Part model, mm, in its own coordinate system. Face numbers are marked on the shaded views. A direction names the side the tool comes from. Round coordinates to 2 decimals unless told otherwise and drop trailing zeros. Order: outer loops, then holes, each group sorted by start corner. A loop starts at its lowest first (then second) coordinate and runs counter-clockwise, first axis right, second up. Notation, with made-up numbers: (53, 73) - (61, 73) arc R28 ccw to (61, 112) - close; hole circle Ø7 at (-3.75, -37). An arc over 180 degrees is marked (long way). Return JSON: item names as keys, results as strings. Group by question number.
Item 1: Saw through at D-D on x = 23.5. List the corners of the cut face in (y, z), and give its area (3 significant figures).
Item 2: Two-plate mould, pull along Y, no slides. Class the marked faces 1, 2 and 3: released by +Y, released by -Y, zero draft, split by the parting line, or undercut.
Item 3: Saw through at A-A on x = -18. List the corners of the cut face in (y, z), and give its area (3 significant figures).
Item 4: Drop flat-ended pins along their axis: pin 1 (1 mm diameter, centred on x = -17.5, z = 6, fed in from -Y); pin 2 (1.5 mm diameter, centred on x = 13, z = 5, fed in from -Y); pin 3 (4 mm diameter, centred on y = -36.5, z = 8, fed in from -X); pin 4 (8 mm diameter, centred on x = 0, y = 57.5, fed in from -Z). Give the stop position or say it passes through.
Item 5: Tool access for the marked faces 4, 5 and 6: list every direction of +Z, -Z, +X, -X, +Y, -Y with a clear straight run to the whole face (end or side of a thin tool).
Item 6: Probe probe 1 along Y at (x, z) = (0, 3); probe 2 along Y at (x, z) = (17, 12); probe 3 along X at (y, z) = (-31.5, 5). List the from-to ranges inside material, lowest first.
Item 7: Saw through at C-C on y = 15.5. List the corners of the cut face in (x, z).
```python
from build123d import *

# Parameters (mm, degrees)
EXTRUDE_1_DEPTH     = 15
SKETCH_6_R          = 3.5
CUT_EXTRUDE_2_DEPTH = 15
SKETCH_7_R          = 10.1
CUT_EXTRUDE_3_DEPTH = 2
SKETCH_8_R          = 0.5
CUT_EXTRUDE_4_DEPTH = 3


with BuildPart() as part:
    # ｽｹｯﾁ1 → ﾎﾞｽ - 押し出し1 (new body)
    with BuildSketch(Plane.XY):
        with BuildLine():
            Line((10.546944731, 68.165925034), (9.641814145, 68.990666647))
            ThreePointArc((9.641814145, 68.990666647), (-9.131421435, 69.400300104), (-13.594616806, 51.160726074))
            Line((-13.594616806, 51.160726074), (4.986432096, 11.313538113))
            ThreePointArc((4.986432096, 11.313538113), (5.221931994, 9.524738795), (4.388829079, 7.924362985))
            Line((4.388829079, 7.924362985), (-40.303464689, -36.767930783))
            ThreePointArc((-40.303464689, -36.767930783), (-41.182112782, -38.903012739), (-40.283913759, -41.029943849))
            ThreePointArc((-40.283913759, -41.029943849), (41.397896806, -39.905690573), (39.524106652, 41.762363359))
            Line((39.524106652, 41.762363359), (37.916838192, 43.226882625))
            Line((37.916838192, 43.226882625), (10.546944731, 68.165925034))
        make_face()
        with BuildLine():
            ThreePointArc((5.093338956, 1.55780505), (7.735603832, 2.390907965), (9.933582661, 0.704339492))
            Line((9.933582661, 0.704339492), (27.046217634, -35.993824637))
            ThreePointArc((27.046217634, -35.993824637), (27.212084573, -38.085077821), (25.967336583, -39.773702754))
            ThreePointArc((25.967336583, -39.773702754), (-1.972837213, -47.459012983), (-29.17877254, -37.481318454))
            ThreePointArc((-29.17877254, -37.481318454), (-30.330146685, -35.299826939), (-29.457223039, -32.992756945))
            Line((-29.457223039, -32.992756945), (5.093338956, 1.55780505))
        make_face(mode=Mode.SUBTRACT)
        with BuildLine():
            ThreePointArc((35.231836325, -31.858557864), (32.560090836, -32.813013733), (30.287744354, -31.114293205))
            Line((30.287744354, -31.114293205), (-2.054746852, 38.244403012))
            ThreePointArc((-2.054746852, 38.244403012), (-1.895310582, 41.077194163), (0.553480425, 42.510214831))
            ThreePointArc((0.553480425, 42.510214831), (5.039223996, 43.371793408), (9.057681155, 45.543478261))
            ThreePointArc((9.057681155, 45.543478261), (10.270904088, 46.091905397), (11.601973614, 46.061309233))
            ThreePointArc((11.601973614, 46.061309233), (45.455779175, 13.784851815), (35.231836325, -31.858557864))
        make_face(mode=Mode.SUBTRACT)
    extrude(amount=EXTRUDE_1_DEPTH)

    # ｽｹｯﾁ6 → ｶｯﾄ - 押し出し2 (cut)
    with BuildSketch(Plane.XY.offset(15)):
        with Locations((0, 57.5)):
            Circle(SKETCH_6_R)
    extrude(amount=-CUT_EXTRUDE_2_DEPTH, mode=Mode.SUBTRACT)

    # ｽｹｯﾁ7 → ｶｯﾄ - 押し出し3 (cut)
    with BuildSketch(Plane.XY.offset(15)):
        with Locations((0, 57.5)):
            Circle(SKETCH_7_R)
    extrude(amount=-CUT_EXTRUDE_3_DEPTH, mode=Mode.SUBTRACT)

    # ｽｹｯﾁ8 → ｶｯﾄ - 押し出し4 (cut)
    with BuildSketch(Plane.XY.offset(13)):
        with Locations((-3.5, 65.5)):
            Circle(SKETCH_8_R)
        with Locations((0, 65.5)):
            Circle(SKETCH_8_R)
        with Locations((3.5, 65.5)):
            Circle(SKETCH_8_R)
        with Locations((8, 57.5)):
            Circle(SKETCH_8_R)
        with Locations((8, 61)):
            Circle(SKETCH_8_R)
        with Locations((8, 54)):
            Circle(SKETCH_8_R)
        with Locations((0, 49.5)):
            Circle(SKETCH_8_R)
        with Locations((3.5, 49.5)):
            Circle(SKETCH_8_R)
        with Locations((-3.5, 49.5)):
            Circle(SKETCH_8_R)
        with Locations((-8, 57.5)):
            Circle(SKETCH_8_R)
        with Locations((-8, 54)):
            Circle(SKETCH_8_R)
        with Locations((-8, 61)):
            Circle(SKETCH_8_R)
    extrude(amount=-CUT_EXTRUDE_4_DEPTH, mode=Mode.SUBTRACT)


solid = part.part
```
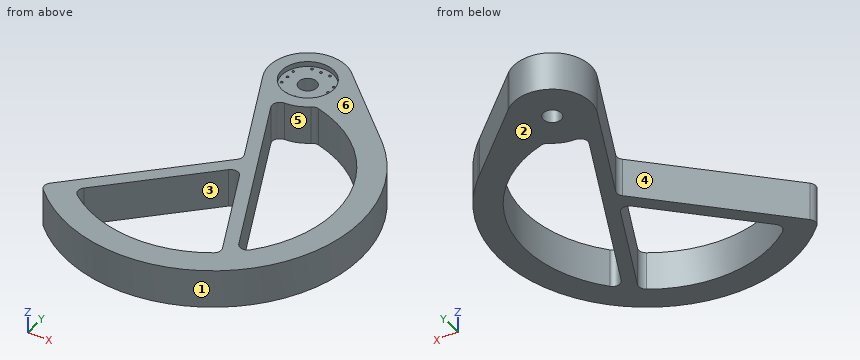
Filled in:
{
 "1": {"outline": "(-52.48, 0) - (-41.28, 0) - (-41.28, 15) - (-52.48, 15) - close; (-28.39, 0) - (-16.56, 0) - (-16.56, 15) - (-28.39, 15) - close; (41.28, 0) - (56.36, 0) - (56.36, 15) - (41.28, 15) - close", "area": "572 mm^2"},
 "2": {"face 1": "split by the parting line", "face 2": "zero draft", "face 3": "undercut"},
 "3": {"outline": "(-54.61, 0) - (-43.96, 0) - (-43.96, 15) - (-54.61, 15) - close; (-21.54, 0) - (-14.46, 0) - (-14.46, 15) - (-21.54, 15) - close", "area": "266 mm^2"},
 "4": {"pin 1": "stops at y = -54.93", "pin 2": "stops at y = -56.18", "pin 3": "stops at x = -41.16", "pin 4": "stops at z = 0"},
 "5": {"face 4": "+Z, -Z, -X", "face 5": "+Z, -Z", "face 6": "+Z, +X, -X, +Y, -Y"},
 "6": {"probe 1": "y = -57.5 to -47.5, -3.54 to 3.54, 22.01 to 33.84, 42.44 to 54, 61 to 72.5", "probe 2": "y = -54.93 to -44.35, -14.45 to -2.62, 44.35 to 62.29", "probe 3": "x = -35.04 to -27.96, 24.95 to 30.5, 35.55 to 48.1"},
 "7": {"outline": "(3.03, 0) - (8.55, 0) - (8.55, 15) - (3.03, 15) - close; (44.9, 0) - (55.37, 0) - (55.37, 15) - (44.9, 15) - close"}
}
